Geometry check sheet. Reference: the model listing, model coordinates, mm. Round coordinates to 2 decimals unless told otherwise and drop trailing zeros. Write each loop counter-clockwise with the first axis right and the second up, starting at its lowest first coordinate (ties: lowest second). Pieces come first, ordered by that corner, then holes. Notation, with made-up numbers: (-27, 36.25) - (-5, 36.25) arc R19 ccw to (-5, 58.25) - close; hole circle Ø7 at (-3.75, 20.5). An arc over 180 degrees is marked (long way). Return JSON: item names as keys, results as strings. Group by question number.
Autodesk Fusion 360 part; units mm, degrees
sketch "Sketch1" plane through (0, 0, 0) normal (0, 0, 1) x (1, 0, 0)
  circle A0 centre (14, 0) radius 2.05
  circle A1 centre (14, 0) radius 3
  circle A2 centre (-14, 0) radius 3
  circle A3 centre (-14, 0) radius 2.05
  line L0 (-14, 3) -> (14, 3)
  line L1 (-14, -3) -> (14, -3)
  line L2 (-14, 0) -> (14, 0) construction
  dimension "d1" = 4.1
  dimension "d2" = 6
  dimension "d3" = 28
  dimension "d4" = 6
  dimension "d5" = 4.1
extrude "Extrude1" add sketch "Sketch1" along normal blind 1
equation "d4 = d2"
equation "d5 = d1"
1. Section check C-C (z = 0.6). Enter the section's corners in (x, y), and give its area (3 significant figures).
2. Section check D-D (x = 13.5). Enter the section's corners in (y, z), and give its area (3 significant figures).
3. Section check B-B (x = -13). Enter the section's corners in (y, z).
4. Material ranges on line 1 along Y through (x, z) = (14, 0.5); line 2 along X through (y, z) = (0.55, 0.3); line 3 along X through (y, z) = (0.65, 0.95), recorded low to high.
5. Mould release check, pull along Y, two halves, no side actions. Record for faces 1 (the face through (0, 0, 1)), 2 (the face through (-0.2, 3, 0.5)), 3 (the face through (-16.05, -0.09, 0.49)): pulls with the +Y half, pulls with the -Y half, needs draft (parallel to the pull), parting line crosses it, or undercut.
6. Depth check by flat-ended pin: pin 1 Ø3.5 at (x, y) = (14, 0) entering from -Z. Enter the tip coordinate at first touch or a pass-through.
7. Section check A-A (y = 0). Enter the section's corners in (x, z), and give its area (3 significant figures).
Result sheet:
{
 "1": {"outline": "(-14, -3) - (14, -3) arc R3 ccw to (14, 3) - (-14, 3) arc R3 ccw to start; hole circle Ø4.1 at (-14, 0); hole circle Ø4.1 at (14, 0)", "area": "170 mm²"},
 "2": {"outline": "(-3, 0) - (-1.99, 0) - (-1.99, 1) - (-3, 1) - close; (1.99, 0) - (3, 0) - (3, 1) - (1.99, 1) - close", "area": "2.02 mm²"},
 "3": {"outline": "(-3, 0) - (-1.79, 0) - (-1.79, 1) - (-3, 1) - close; (1.79, 0) - (3, 0) - (3, 1) - (1.79, 1) - close"},
 "4": {"line 1": "y = -3 to -2.05, 2.05 to 3", "line 2": "x = -16.95 to -15.97, -12.03 to 12.03, 15.97 to 16.95", "line 3": "x = -16.93 to -15.94, -12.06 to 12.06, 15.94 to 16.93"},
 "5": {"face 1": "needs draft", "face 2": "pulls with the +Y half", "face 3": "undercut"},
 "6": {"pin 1": "passes through"},
 "7": {"outline": "(-17, 0) - (-16.05, 0) - (-16.05, 1) - (-17, 1) - close; (-11.95, 0) - (11.95, 0) - (11.95, 1) - (-11.95, 1) - close; (16.05, 0) - (17, 0) - (17, 1) - (16.05, 1) - close", "area": "25.8 mm²"}
}
